Geometry: final body of the model. Coordinates: model frame, mm. A direction names the side the tool comes from. Give positions to 0.01 mm unless a question says otherwise; leave off trailing zeros. Write each loop counter-clockwise with the first axis right and the second up, starting at its lowest first coordinate (ties: lowest second). Pieces come first, ordered by that corner, then holes. Notation, with made-up numbers: (-30, -10) -> (10, -10) arc R18 cw to (10, -4) -> close; hole circle Ø7 at (81, 29). An arc over 180 degrees is marked (long way). Answer as a JSON object with one key per item and string values. Group by question number.
(1) Section query B-B on y = -19. Output: boundary loops of the cut face in (x, z).
(2) Draft query along Y for faces 4 (the face through (15.105, -2.26, 9.197)), 5 (the face through (11.8, -0.5, -4.5)), 6 (the face through (12, -3.9, 3)). Return one class per face: +Y half, -Y half, draft (parallel to the pull), parting line (faces both ways), or undercut.
(3) Section query A-A on x = 12. Output: boundary loops of the cut face in (y, z), plus the area to 3 significant figures.
(4) Set-up query: faces 1 (the face through (12, -3.6, 3.5)), 2 (the face through (12.1, -28.4, 3.5)), 3 (the face through (20, -21, 1.5)). Return all of +Z, -Z, +X, -X, +Y, -Y with unobstructed straight access to the full face (end or side cutting, diameter ignored); none if empty.
(5) Section query C-C on z = 3. Output: boundary loops of the cut face in (x, y), plus the area to 3 significant figures.
(6) Section query D-D on z = -2.25. Output: boundary loops of the cut face in (x, y), plus the area to 3 significant figures.
(7) Material intervals for probe 1 along X at (y, z) = (-16, -2.25); probe 2 along Z at (x, y) = (6.5, -2.45); probe 3 along X at (y, z) = (-5, 9.75), sorted ascending.
(8) Contact query for flat-ended pins moving along their axis: pin 1 Ø5 at (x, y) = (11, -23) entering from +Z; pin 2 Ø2.5 at (x, z) = (10.5, 6) entering from -Y; pin 3 Ø3 at (x, z) = (6, 5.5) entering from -Y. Output: stop coordinate, or through.
from build123d import *

# Parameters (mm, degrees)
F0_W           = 24
F0_H           = 12
F1_DEPTH       = 3
F3_D           = 3
F3_CBORE_D     = 6.5
F3_CBORE_DEPTH = 1.5
F4_DEPTH       = 26
F7_R           = 4
F8_R           = 9.25
F9_DEPTH       = 25
F10_DEPTH      = 5
F11_DEPTH      = 2
F2_W           = 2
F2_H           = 8.5
F12_REACH      = 34.7331245983
F5_W           = 2
F5_H           = 8.5
F13_REACH      = 34.7331245983
F14_SIZE       = 1
F15_R          = 2
F17_DEPTH      = 25


# Not quite as in the source:
# - a feature names something its author has since deleted; it is built from what else it names


with BuildPart() as f1:
    # F0 (on Front) → F1 (new body)
    with BuildSketch(Plane.XZ):
        with Locations((12, 6)):
            Rectangle(F0_W, F0_H)
    extrude(amount=F1_DEPTH)

    # F3 (through all)
    with Locations(Plane.XZ.offset(3)):
        with Locations((6.5, 7), (17.5, 7)):
            CounterBoreHole(F3_D / 2, F3_CBORE_D / 2, F3_CBORE_DEPTH)

    # F2 (on face) → F4 (join)
    with BuildSketch(Plane.XZ.offset(3)):
        Polygon((0, 3.5), (0, 0), (24, 0), (24, 3.5), (22, 3.5), (2, 3.5), align=None)
    extrude(amount=F4_DEPTH)

    # F7
    f7_edges = [f1.edges().sort_by_distance(p)[0] for p in [
        (24, -29, 1.75),
        (0, -29, 1.75),
    ]]
    fillet(f7_edges, radius=F7_R)

    # F8 (on face) → F9 (cut)
    with BuildSketch(Plane(origin=(0, 0, 0), x_dir=(1, 0, 0), z_dir=(0, 0, -1))):
        with Locations((12, 16)):
            Circle(F8_R)
    extrude(amount=-F9_DEPTH, mode=Mode.SUBTRACT)

    # F10 (add): a face of the model
    f10_faces = [f1.faces().sort_by_distance(p)[0] for p in [
        (0.3764306045, -12.5, 0),
    ]]
    extrude(f10_faces, amount=F10_DEPTH)

    # F6 (on face) → F11 (cut)
    with BuildSketch(Plane.XY.offset(3.5)):
        Polygon((0, -19.4153903092), (5.0140617428, -28.1), (18.9859382572, -28.1), (24, -19.4153903092), (24, -12.5846096908), (18.9859382572, -3.9), (5.0140617428, -3.9), (0, -12.5846096908), align=None)
    extrude(amount=-F11_DEPTH, mode=Mode.SUBTRACT)

    f12_end = Plane(origin=(2.5070308714, -8.2423048454, 2.5), x_dir=(0.5, 0.8660254038, 0), z_dir=(0.8660254038, -0.5, 0))
    # F2 (on face) → F12 (join, up to a plane its end follows)
    with BuildSketch(Plane.XZ.offset(3)):
        with Locations((1, 7.75)):
            Rectangle(F2_W, F2_H)
    f12_long = extrude(amount=F12_REACH, mode=Mode.PRIVATE)
    add(split(f12_long, bisect_by=f12_end, keep=Keep.BOTTOM, mode=Mode.PRIVATE))

    f13_end = Plane(origin=(21.4929691286, -8.2423048454, 2.5), x_dir=(0.5, -0.8660254038, 0), z_dir=(-0.8660254038, -0.5, 0))
    # F5 (on face) → F13 (join, up to a plane its end follows)
    with BuildSketch(Plane.XZ.offset(3)):
        with Locations((23, 7.75)):
            Rectangle(F5_W, F5_H)
    f13_long = extrude(amount=F13_REACH, mode=Mode.PRIVATE)
    add(split(f13_long, bisect_by=f13_end, keep=Keep.BOTTOM, mode=Mode.PRIVATE))

    # F14
    f14_edges = [f1.edges().sort_by_distance(p)[0] for p in [
        (12, 0, -5),
    ]]
    chamfer(f14_edges, length=F14_SIZE)

    # F15
    f15_edges = [f1.edges().sort_by_distance(p)[0] for p in [
        (24, -6.292305, 12),
        (0, -6.292305, 12),
    ]]
    fillet(f15_edges, radius=F15_R)

    # F16 (on face) → F17 (cut)
    with BuildSketch(Plane.YZ.offset(24)):
        Polygon((-12.5846096908, 12), (-12.5846096908, 1.5), (-3, 12), align=None)
    extrude(amount=-F17_DEPTH, mode=Mode.SUBTRACT)


solid = f1.part
Answer list:
{
 "1": {"outline": "(0, -5) -> (3.25, -5) -> (3.25, 1.5) -> (0, 1.5) -> close; (20.75, -5) -> (24, -5) -> (24, 1.5) -> (20.75, 1.5) -> close"},
 "2": {"face 4": "draft", "face 5": "+Y half", "face 6": "undercut"},
 "3": {"outline": "(-29, -5) -> (-25.25, -5) -> (-25.25, 1.5) -> (-28.1, 1.5) -> (-28.1, 3.5) -> (-29, 3.5) -> close; (-6.75, -5) -> (-1, -5) -> (0, -4) -> (0, 12) -> (-3, 12) -> (-3, 3.5) -> (-3.9, 3.5) -> (-3.9, 1.5) -> (-6.75, 1.5) -> close", "area": "103 mm2"},
 "4": {"face 1": "+Z, -Y", "face 2": "+Z, +X, -X, -Y", "face 3": "+Z"},
 "5": {"outline": "(0, -25) arc R4 ccw to (4, -29) -> (20, -29) arc R4 ccw to (24, -25) -> (24, -19.42) -> (18.99, -28.1) -> (5.01, -28.1) -> (0, -19.42) -> close; (0, -11.22) -> (0.79, -11.22) -> (5.01, -3.9) -> (18.99, -3.9) -> (23.21, -11.22) -> (24, -11.22) -> (24, 0) -> (0, 0) -> close", "area": "194 mm2"},
 "6": {"outline": "(0, -25) arc R4 ccw to (4, -29) -> (20, -29) arc R4 ccw to (24, -25) -> (24, 0) -> (0, 0) -> close; hole circle Ø18.5 at (12, -16)", "area": "420 mm2"},
 "7": {"probe 1": "0 to 2.75, 21.25 to 24", "probe 2": "-5 to 3.75, 10.25 to 12", "probe 3": "0 to 2, 22 to 24"},
 "8": {"pin 1": "z = 1.5", "pin 2": "y = -3", "pin 3": "y = -1.5"}
}
